Build history of the part. All positions in model axes, mm. Round coordinates to 2 decimals unless told otherwise and drop trailing zeros. Loops run counter-clockwise (first coordinate to the right, second up) from the corner with the lowest first, then second, coordinate; pieces in that order, holes last. Notation, with made-up numbers: M 76,-35.75 L 95,-35.75 A7 cw 95,-23.75 Z; hole C 17,26 d9. An arc over 180 degrees is marked long. Use one line per item in the form item = value. Start each with the question number.
```python
from build123d import *

# Parameters (mm, degrees)
SKETCH_1_R          = 1.45
EXTRUDE_1_DEPTH     = 2
CUT_EXTRUDE_1_DEPTH = 70.491006612
FILLET_1_R          = 3


with BuildPart() as part:
    # 草图1 → 凸台-拉伸1 (new body)
    with BuildSketch(Plane(origin=(0, 0, 0), x_dir=(1, 0, 0), z_dir=(0, 1, 0))):
        Polygon((0, 15), (0, 0), (30, -20), (45, -20), (60, 0), (60, 15), (45, 15), (32, 15), (15, 35), (0, 35), align=None)
        Polygon((30, -16.394448725), (5.408326913, 0), (30, 0), align=None, mode=Mode.SUBTRACT)
        with Locations(Location((37.5, -15, 0), (0, 0, 270))):
            Circle(SKETCH_1_R, mode=Mode.SUBTRACT)
        Polygon((45, 0), (56.25, 0), (45, -15), align=None, mode=Mode.SUBTRACT)
        with Locations(Location((37.5, -5, 0), (0, 0, 270))):
            Circle(SKETCH_1_R, mode=Mode.SUBTRACT)
        with Locations(Location((10, 7.5, 0), (0, 0, 270))):
            Circle(SKETCH_1_R, mode=Mode.SUBTRACT)
        with Locations(Location((7.5, 20, 0), (0, 0, 270))):
            Circle(SKETCH_1_R, mode=Mode.SUBTRACT)
        with Locations(Location((7.5, 30, 0), (0, 0, 270))):
            Circle(SKETCH_1_R, mode=Mode.SUBTRACT)
        Polygon((15, 28.82380953), (26.750238101, 15), (15, 15), align=None, mode=Mode.SUBTRACT)
        with Locations(Location((30, 7.5, 0), (0, 0, 270))):
            Circle(SKETCH_1_R, mode=Mode.SUBTRACT)
        with Locations(Location((50, 7.5, 0), (0, 0, 270))):
            Circle(SKETCH_1_R, mode=Mode.SUBTRACT)
    extrude(amount=EXTRUDE_1_DEPTH)

    # 草图2 → 切除-拉伸1 (cut, through all)
    with BuildSketch(Plane(origin=(0, 2, 0), x_dir=(1, 0, 0), z_dir=(0, 1, 0))):
        Polygon((15, 35), (15, 15), (32, 15), align=None)
    extrude(amount=-CUT_EXTRUDE_1_DEPTH, mode=Mode.SUBTRACT)

    # 圆角1
    fillet_1_edges = [part.edges().sort_by_distance(p)[0] for p in [
        (15, 1, -15),
        (45, 1, 15),
        (56.25, 1, 0),
        (45, 1, 0),
        (30, 1, 0),
        (5.408326913, 1, 0),
        (30, 1, 16.394448725),
        (60, 1, -15),
        (60, 1, 0),
        (45, 1, 20),
        (30, 1, 20),
        (0, 1, 0),
        (0, 1, -35),
        (15, 1, -35),
    ]]
    fillet(fillet_1_edges, radius=FILLET_1_R)


solid = part.part
```
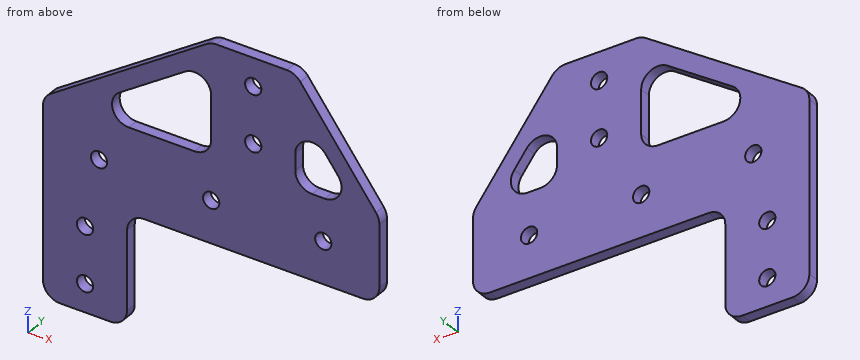
Q1. Saw through at C-C (z = -7.5). Give the cut face in (x, y), and give its area (3 significant figures).
Q2. Saw through at A-A (x = 37.5). Give the cut face in (y, z).
Q3. Saw through at B-B (z = 15). Give the cut face in (x, y).
Q4. Wall check: probe 1 along X at (y, z) = (1.35, -7.5); probe 2 along X at (y, z) = (1.35, -30); probe 3 along X at (y, z) = (1.75, 2). Give the ranges that are in metal, low to high.
Q5. Drop flat-ended pins along their axis: P1, Ø2.5, axis at x = 30, z = -7.5, coming from the +Y side; P2, Ø0.6, axis at x = 37, y = 0.5, coming from the -Z side; P3, Ø1, axis at x = 49.5, y = 1, coming from the +Z side. Give the stop position or say it passes through.
Q6. Saw through at D-D (x = 7.5). Give the cut face in (y, z).
Filled in:
q1.outline = M 0,0 L 8.55,0 L 8.55,2 L 0,2 Z; M 11.45,0 L 28.55,0 L 28.55,2 L 11.45,2 Z; M 31.45,0 L 48.55,0 L 48.55,2 L 31.45,2 Z; M 51.45,0 L 60,0 L 60,2 L 51.45,2 Z
q1.area = 103 mm²
q2.outline = M 0,-15 L 2,-15 L 2,3.55 L 0,3.55 Z; M 0,6.45 L 2,6.45 L 2,13.55 L 0,13.55 Z; M 0,16.45 L 2,16.45 L 2,20 L 0,20 Z
q3.outline = M 22.5,0 L 36.05,0 L 36.05,2 L 22.5,2 Z; M 38.95,0 L 48.75,0 L 48.75,2 L 38.95,2 Z
q4.probe_1 = 0 to 8.55, 11.45 to 28.55, 31.45 to 48.55, 51.45 to 60
q4.probe_2 = 0 to 6.05, 8.95 to 15
q4.probe_3 = 3 to 12.49, 29.83 to 45.17, 53.08 to 58.5
q5.P1 = through
q5.P2 = -15
q5.P3 = 14.67
q6.outline = M 0,-35 L 2,-35 L 2,-31.45 L 0,-31.45 Z; M 0,-28.55 L 2,-28.55 L 2,-21.45 L 0,-21.45 Z; M 0,-18.55 L 2,-18.55 L 2,5 L 0,5 Z
